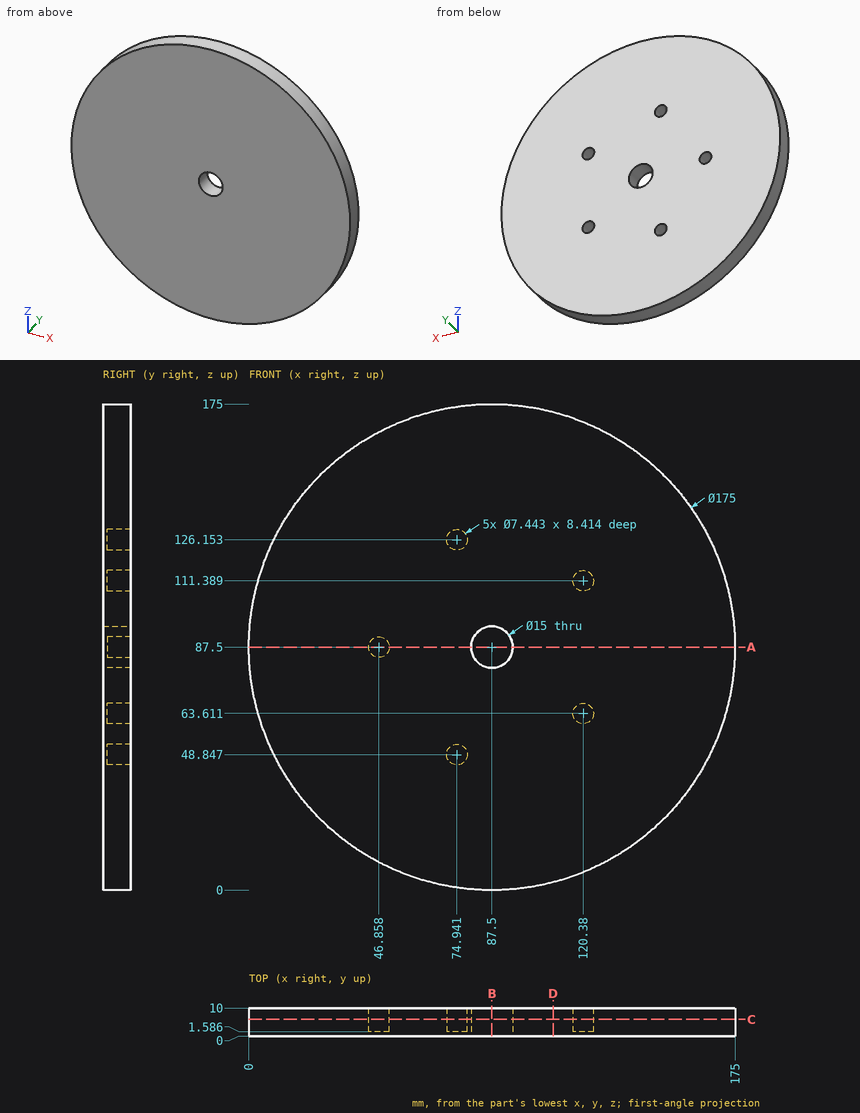
Can you work these out from the drawing? Everything is in mm from the part's minimum corner. Round coordinates to 2 decimals unless told otherwise and drop trailing zeros. Loops run counter-clockwise (first coordinate to the right, second up) from the corner with the lowest first, then second, coordinate; pieces in that order, holes last. Notation, with made-up numbers: (45, -22.5) - (92, -22.5) arc R25 ccw to (92, 9.5) - close; hole circle Ø6 at (39, -25.5). An arc over 180 degrees is marked (long way). One line per question, with ' | ' between items. Start each with the question number.
Q1. I want a section at B-B (x = 87.5). Write out the boundary of the cut face in (y, z), then the cut area to 3 significant figures.
Q2. Will these pins go through, and if not, where does the flat tip stop? pin 1 (1 mm diameter, centred on x = 99.5, y = 1.5, fed in from -Z); pin 2 (3.5 mm diameter, centred on x = 119, z = 62.5, fed in from +Y); pin 3 (3 mm diameter, centred on y = 4, z = 60.5, fed in from +X).
Q3. I want a section at D-D (x = 109.5). Write out the boundary of the cut face in (y, z), then the cut area to 3 significant figures.
Q4. I want a section at A-A (z = 87.5). Write out the boundary of the cut face in (x, y).
Q5. I want a section at C-C (y = 6). Write out the boundary of the cut face in (x, z), then the cut area to 3 significant figures.
Q6. Please list where these lines run through material, in increasing order: line 1 (X direction, y = 7, z = 87.5); line 2 (Z direction, x = 47, y = 6.75); line 3 (Z direction, x = 47.5, y = 6.5) (1 decimal). Write a range as [from, to].
Response values:
1) outline: (0, 0) - (10, 0) - (10, 80) - (0, 80) - close; (0, 95) - (10, 95) - (10, 175) - (0, 175) - close | area: 1,600 mm²
2) pin 1: stops at z = 0.76 | pin 2: stops at y = 1.59 | pin 3: stops at x = 171.2
3) outline: (0, 2.81) - (10, 2.81) - (10, 172.19) - (0, 172.19) - close | area: 1,690 mm²
4) outline: (0, 0) - (80, 0) - (80, 10) - (50.58, 10) - (50.58, 1.59) - (43.14, 1.59) - (43.14, 10) - (0, 10) - close; (95, 0) - (175, 0) - (175, 10) - (95, 10) - close
5) outline: circle Ø175 at (87.5, 87.5); hole circle Ø7.44 at (46.86, 87.5); hole circle Ø7.44 at (74.94, 48.85); hole circle Ø7.44 at (74.94, 126.15); hole circle Ø15 at (87.5, 87.5); hole circle Ø7.44 at (120.38, 63.61); hole circle Ø7.44 at (120.38, 111.39) | area: 23,700 mm²
6) line 1: x = [0, 43.14], [50.58, 80], [95, 175] | line 2: z = [9.94, 83.78], [91.22, 165.06] | line 3: z = [9.7, 83.8], [91.2, 165.3]
